Geometry check sheet. Reference: the model listing, model coordinates, mm. Face numbers are marked on the shaded views. A direction names the side the tool comes from. Give positions to 0.01 mm unless a question says otherwise; leave off trailing zeros. Loops run counter-clockwise (first coordinate to the right, second up) from the corner with the lowest first, then second, coordinate; pieces in that order, holes last.
1. Cross-section at C-C, the plane x = 35. Record the cut outline in (y, z), plus the area to 3 significant figures.
2. Cross-section at A-A, the plane x = 10. Record the cut outline in (y, z), plus the area to 3 significant figures.
3. Go/stop test with flat-tipped pins: pin 1 Ø4 at (x, z) = (38, -16.5) entering from +Y; pin 2 Ø12 at (y, z) = (-2.5, -9.5) entering from -X; pin 3 Ø1.5 at (x, z) = (11, -12) entering from -Y; pin 4 Ø1 at (x, z) = (20.5, -4) entering from +Y. Record where each tip stops, or that it passes through.
4. Tool access check on the marked faces 1, 2 and 3. Record the directions out of +Z, -Z, +X, -X, +Y, -Y that give a thin tool (end or side, any length) a straight path to the whole face; none if there is none.
5. Material ranges on L1, parallel to Z at x = 10.5, y = -2.5; L2, parallel to Y at x = 5, z = -3; L3, parallel to Y at x = 35, z = -10, recorded low to high.
6. Release check for a two-part mould opening along Y. For the marked faces 4, 5 and 6 record: +Y half, -Y half, draft (parallel to the pull), parting line (faces both ways), or undercut.
7. Cross-section at D-D, the plane z = -17.5. Record the cut outline in (x, y).
8. Cross-section at B-B, the plane z = -10. Record the cut outline in (x, y), plus the area to 3 significant figures.
from build123d import *

# Parameters (mm, degrees)
EXTRUDE_1_DEPTH     = 20
FILLET_1_RADIUS     = 10
FILLET_1_LENGTH     = 11.313708499
SKETCH_4_R          = 6
CUT_EXTRUDE_1_DEPTH = 60.222889557
CUT_EXTRUDE_2_DEPTH = 65.213321417


with BuildPart() as part:
    # 草图1 → 凸台-拉伸1 (new body)
    with BuildSketch(Plane.XY):
        Polygon((0, 0), (28, 0), (49.213203436, 21.213203436), (57.213203436, 13.213203436), (36, -8), (0, -8), align=None)
    extrude(amount=-EXTRUDE_1_DEPTH)

    # 圆角1: full round fillet: the end face becomes a half cylinder, R = half its width
    fillet_1_face = Plane((53.213203436, 17.213203436, -10), x_dir=(-0.707106781187, 0.707106781187, 0), z_dir=(0.707106781187, 0.707106781187, 0))  # on the end face: x along it, z out of the body
    fillet_1_slab = fillet_1_face.offset(-FILLET_1_RADIUS / 2) * Box(FILLET_1_LENGTH, 2 * FILLET_1_RADIUS, FILLET_1_RADIUS, mode=Mode.PRIVATE)  # the body's end, R deep
    fillet_1_round = Plane((46.142135624, 10.142135624, -10), x_dir=(0.707106781187, 0.707106781187, 0), z_dir=(-0.707106781187, 0.707106781187, 0)) * Cylinder(FILLET_1_RADIUS, FILLET_1_LENGTH, mode=Mode.PRIVATE)  # its axis R under the face
    add(fillet_1_slab - fillet_1_round, mode=Mode.SUBTRACT)

    # 草图4 → 切除-拉伸1 (cut, through all)
    with BuildSketch(Plane(origin=(14, -14, 0), x_dir=(0, 0, 1), z_dir=(-0.7071067811865488, 0.7071067811865462, 0))):
        with Locations(Location((-10, 39.798989873, 0), (0, 0, 270))):
            Circle(SKETCH_4_R)
    extrude(amount=-CUT_EXTRUDE_1_DEPTH, mode=Mode.SUBTRACT)

    # 草图2 → 切除-拉伸2 (cut, through all)
    with BuildSketch(Plane(origin=(0, 0, 0), x_dir=(1, 0, 0), z_dir=(0, 1, 0))):
        with BuildLine():
            Line((7, 6.5), (23, 6.5))
            ThreePointArc((23, 6.5), (26.5, 10), (23, 13.5))
            Line((23, 13.5), (7, 13.5))
            ThreePointArc((7, 13.5), (3.5, 10), (7, 6.5))
        make_face()
    extrude(amount=-CUT_EXTRUDE_2_DEPTH, mode=Mode.SUBTRACT)


solid = part.part
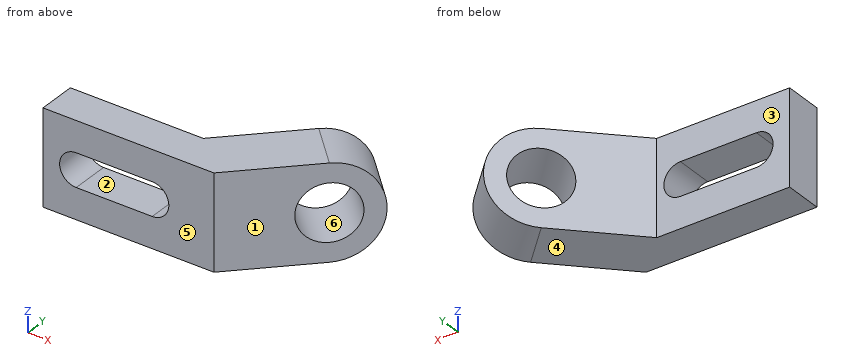
Result:
1. outline: (-8, -20) - (7, -20) - (7, 0) - (-8, 0) - close
1. area: 300 mm2
2. outline: (-8, -20) - (0, -20) - (0, -13.5) - (-8, -13.5) - close; (-8, -6.5) - (0, -6.5) - (0, 0) - (-8, 0) - close
2. area: 104 mm2
3. pin 1: stops at y = 12
3. pin 2: stops at x = 0
3. pin 3: passes through
3. pin 4: stops at y = 0
4. face 1: +Z, -Z, +X, -Y
4. face 2: +Y, -Y
4. face 3: +Z, -Z, -X, +Y
5. L1: z = -20 to -13.5, -6.5 to 0
5. L2: y = -8 to 0
5. L3: y = -8 to 7
6. face 4: draft
6. face 5: -Y half
6. face 6: undercut
7. outline: (0, -8) - (36, -8) - (54.82, 10.82) - (46.82, 18.82) - (28, 0) - (0, 0) - close
8. outline: (0, -8) - (3.5, -8) - (3.5, 0) - (0, 0) - close; (26.5, -8) - (36, -8) - (45.9, 1.9) - (37.9, 9.9) - (28, 0) - (26.5, 0) - close; (46.38, 18.38) - (54.38, 10.38) - (57.21, 13.21) - (49.21, 21.21) - close
8. area: 276 mm2
